The model under review builds one solid part; all positions refer to its coordinate system, in mm. Face numbers are marked on the shaded views. A direction names the side the tool comes from. Coordinates: 2 decimals unless noted, no trailing zeros. Write each loop counter-clockwise with the first axis right and the second up, starting at its lowest first coordinate (ties: lowest second). Pieces come first, ordered by that corner, then holes.
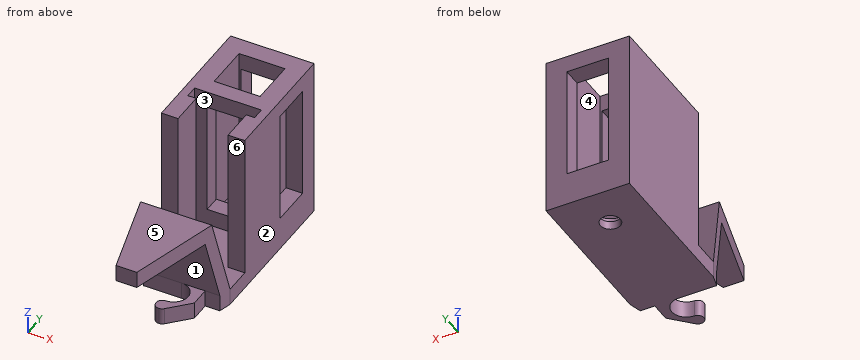
```python
from build123d import *

# Parameters (mm, degrees)
SKETCH002_W             = 50
SKETCH002_H             = 20
PAD001_DEPTH            = 4
SKETCH003_R             = 4
POCKET001_DEPTH         = 2
SKETCH004_R             = 2.4
POCKET002_DEPTH         = 2
SKETCH016_W             = 11
SKETCH016_H             = 11
SKETCH016_W_2           = 33
SKETCH016_H_2           = 20
PAD007_DEPTH            = 35
SKETCH017_W             = 10
SKETCH017_H             = 27
POCKET009_DEPTH         = 20
SKETCH018_W             = 10
SKETCH018_H             = 27
POCKET010_DEPTH         = 4
POCKET011_DEPTH         = 20
POCKET016_DEPTH         = 25
POCKET017_DEPTH         = 4
POCKET018_DEPTH         = 4
BODY002_PLACEMENT_ANGLE = 90.0000000001


with BuildPart() as part:
    # Sketch002 (on Face1 of CopyPocket) → Pad001 (new body)
    with BuildSketch(Plane.XY.offset(8)):
        with Locations((-15, 0)):
            Rectangle(SKETCH002_W, SKETCH002_H)
    extrude(amount=PAD001_DEPTH)

    # Sketch003 (on Face6 of Pad001) → Pocket001 (cut)
    with BuildSketch(Plane.XY.offset(12)):
        Circle(SKETCH003_R)
    extrude(amount=-POCKET001_DEPTH, mode=Mode.SUBTRACT)

    # Sketch004 (on Face8 of Pocket001) → Pocket002 (cut)
    with BuildSketch(Plane.XY.offset(10)):
        Circle(SKETCH004_R)
    extrude(amount=-POCKET002_DEPTH, mode=Mode.SUBTRACT)

    # Sketch016 (on Face5 of Pocket002) → Pad007 (join)
    with BuildSketch(Plane.XY.offset(12)):
        Polygon((10, -10), (10, 10), (-20.5, 10), (-20.5, 6), (-12.5, 6), (-12.5, 8), (-9.5, 8), (-9.5, -8), (-12.5, -8), (-12.5, -6), (-20.5, -6), (-20.5, -10), align=None)
        Rectangle(SKETCH016_W, SKETCH016_H, mode=Mode.SUBTRACT)
        with Locations((-43.5, 0)):
            Rectangle(SKETCH016_W_2, SKETCH016_H_2)
    extrude(amount=PAD007_DEPTH)

    # Sketch017 (on Face7 of Pad007) → Pocket009 (cut)
    with BuildSketch(Plane.YZ.offset(10)):
        with Locations((0, 29.5)):
            Rectangle(SKETCH017_W, SKETCH017_H)
    extrude(amount=-POCKET009_DEPTH, mode=Mode.SUBTRACT)

    # Sketch018 (on Face10 of Pocket009) → Pocket010 (cut)
    with BuildSketch(Plane.XZ.offset(10)):
        with Locations((0, 29.5)):
            Rectangle(SKETCH018_W, SKETCH018_H)
    extrude(amount=-POCKET010_DEPTH, mode=Mode.SUBTRACT)

    # Sketch019 (on Face8 of Pocket010) → Pocket011 (cut)
    with BuildSketch(Plane.XZ.offset(10)):
        Polygon((-27, 12), (-32.3589838486, 32), (-54.2871870789, 32), (-54.2871870789, 28), (-34.2871870789, 28), (-30, 12), (-40, 12), (-60, 12), (-60, 47), (-27, 47), align=None)
    extrude(amount=-POCKET011_DEPTH, mode=Mode.SUBTRACT)

    # Sketch027 (on Face22 of Pocket011) → Pocket016 (cut)
    with BuildSketch(Plane.XY.offset(32)):
        Polygon((-54.2871870789, -10), (-54.2871870789, -2.5), (-27, -10), align=None)
        Polygon((-54.2871870789, 2.5), (-54.2871870789, 10), (-27, 10), align=None)
    extrude(amount=-POCKET016_DEPTH, mode=Mode.SUBTRACT)

    # Sketch028 (on Face1 of Pocket016) → Pocket017 (cut)
    with BuildSketch(Plane(origin=(0, 0, 8), x_dir=(1, 0, 0), z_dir=(0, 0, -1))):
        with BuildLine():
            Line((-39.5440001666, 1.0770625108), (-34.8, 5.6754371773))
            Line((-34.8, 5.6754371773), (-30, 5.6754371773))
            Line((-30, 5.6754371773), (-30, 9.1754371773))
            Line((-30, 9.1754371773), (-40, 6.4268944352))
            Line((-40, 0), (-40, 6.4268944352))
            ThreePointArc((-39.5440001666, 1.0770625108), (-39.8813037772, 0.5848075539), (-40, 0))
        make_face()
    extrude(amount=-POCKET017_DEPTH, mode=Mode.SUBTRACT)

    # Sketch029 (on Face1 of Pocket017) → Pocket018 (cut)
    with BuildSketch(Plane(origin=(0, 0, 8), x_dir=(1, 0, 0), z_dir=(0, 0, -1))):
        with BuildLine():
            ThreePointArc((-40, 0), (-38.5, -1.5), (-37, 0))
            ThreePointArc((-30, 0), (-33.5, 3.5), (-37, 0))
            Line((-30, -9.1754371773), (-30, 0))
            Line((-40, -6.4268944352), (-30, -9.1754371773))
            Line((-40, 0), (-40, -6.4268944352))
        make_face()
    extrude(amount=-POCKET018_DEPTH, mode=Mode.SUBTRACT)


with BuildPart() as part_1:
    # Body002 placement: moved
    add(part.part.rotate(Axis((0, 0, 0), (0, 0, 1)), BODY002_PLACEMENT_ANGLE))


solid = part_1.part
```
Item 1: Take a section at B-B, the plane z = 19. Count the separate pieces of the cut face and the enclosed holes in it, plus the area to 3 significant figures.
Solved:
separate pieces: 3
enclosed holes: 0
area: 274 mm2
Item 2: Take a section at D-D, the plane y = -46. Write out the cut boundary in (x, z).
Solved:
outline: (-4.78, 28) - (4.78, 28) - (4.78, 32) - (-4.78, 32) - close
Item 3: For pin 1 (6 mm diameter, centred on y = -42, z = 34, fed in from +X); pin 2 (1 mm diameter, centred on x = 0, z = 17.5, fed in from -Y); pin 3 (2 mm diameter, centred on x = -5.5, z = 10.5, fed in from -Y), all flat-tipped, find the tip position at first contact; note any pin that passes through.
Solved:
pin 1: stops at x = 6.49
pin 2: stops at y = -31.61
pin 3: stops at y = -30
Item 4: Machinability: for the marked faces 4, 5 and 6, which of the approach directions +Z, -Z, +X, -X, +Y, -Y give a long, thin tool a straight path to every point of the face, cutting with its end or side? Answer none if there is none.
Solved:
face 4: +Z
face 5: +Z, +X, -X, -Y
face 6: +Z, +X, -X
Item 5: To check wall thickness, follow line 1 along Y through (x, z) = (7, 40); line 2 along X through (y, z) = (0, 9); line 3 along Y through (x, z) = (-0.5, 12.5). State the ranges of each line that lie inside material, in increasing order.
Solved:
line 1: y = -20.5 to -12.5, -9.5 to -5, 5 to 10
line 2: x = -10 to -2.4, 2.4 to 10
line 3: y = -30.13 to -27.13, -9.5 to -5.5, 5.5 to 10
Item 6: Take a section at C-C, the plane y = -38.5. Write out the cut boundary in (x, z).
Solved:
outline: (-6.84, 28) - (6.84, 28) - (6.84, 32) - (-6.84, 32) - close; (-1.5, 8) - (2.09, 8) - (2.09, 12) - (-1.5, 12) - close
Item 7: Mouldability with a two-part tool opening along Y and no side actions: class the marked faces 1, 2 and 3 as pulls with the +Y half, pulls with the -Y half, needs draft (parallel to the pull), parting line crosses it, or undercut.
Solved:
face 1: pulls with the -Y half
face 2: needs draft
face 3: undercut
Item 8: Take a section at A-A, the plane y = 0. Write out the cut boundary in (x, z).
Solved:
outline: (-10, 8) - (-2.4, 8) - (-2.4, 10) - (-4, 10) - (-4, 12) - (-5.5, 12) - (-5.5, 47) - (-10, 47) - close; (2.4, 8) - (10, 8) - (10, 16) - (6, 16) - (6, 43) - (10, 43) - (10, 47) - (5.5, 47) - (5.5, 12) - (4, 12) - (4, 10) - (2.4, 10) - close
